```python
from build123d import *

# Parameters (mm, degrees)
F1_DEPTH = 12
F3_R     = 3


with BuildPart() as f1:
    # F0 (on Front) → F1 (new body)
    with BuildSketch(Plane.XZ):
        with BuildLine():
            Line((813.389391, 66.97586), (-386.610609, 66.97586))
            Line((-386.610609, 66.97586), (-386.610609, 26.97586))
            Line((-386.610609, 26.97586), (-406.610609, 26.97586))
            Line((-406.610609, 26.97586), (-406.610609, 11.97586))
            ThreePointArc((-406.610609, 11.97586), (-399.288279, -5.70181), (-381.610609, -13.02414))
            Line((-381.610609, -13.02414), (333.389391, -13.02414))
            ThreePointArc((333.389391, -13.02414), (351.06706, -5.70181), (358.389391, 11.97586))
            Line((358.389391, 11.97586), (658.389391, 11.97586))
            ThreePointArc((658.389391, 11.97586), (665.711721, -5.70181), (683.389391, -13.02414))
            Line((683.389391, -13.02414), (808.389391, -13.02414))
            ThreePointArc((808.389391, -13.02414), (826.06706, -5.70181), (833.389391, 11.97586))
            Line((833.389391, 11.97586), (833.389391, 26.97586))
            Line((833.389391, 26.97586), (813.389391, 26.97586))
            Line((813.389391, 26.97586), (813.389391, 66.97586))
        make_face()
    extrude(amount=F1_DEPTH)

    # F3
    f3_edges = [f1.edges().sort_by_distance(p)[0] for p in [
        (213.389391, -12, 66.97586),
        (-386.610609, -12, 46.97586),
        (-396.610609, -12, 26.97586),
        (-406.610609, -12, 19.47586),
        (-399.288279, -12, -5.70181),
        (-24.110609, -12, -13.02414),
        (351.06706, -12, -5.70181),
        (508.389391, -12, 11.97586),
        (665.711721, -12, -5.70181),
        (745.889391, -12, -13.02414),
        (826.06706, -12, -5.70181),
        (833.389391, -12, 19.47586),
        (823.389391, -12, 26.97586),
        (813.389391, -12, 46.97586),
        (213.389391, 0, 66.97586),
        (-386.610609, 0, 46.97586),
        (-396.610609, 0, 26.97586),
        (-406.610609, 0, 19.47586),
        (-399.288279, 0, -5.70181),
        (-24.110609, 0, -13.02414),
        (351.06706, 0, -5.70181),
        (508.389391, 0, 11.97586),
        (665.711721, 0, -5.70181),
        (745.889391, 0, -13.02414),
        (826.06706, 0, -5.70181),
        (833.389391, 0, 19.47586),
        (823.389391, 0, 26.97586),
        (813.389391, 0, 46.97586),
    ]]
    fillet(f3_edges, radius=F3_R)


solid = f1.part
```
The model under review builds one solid part; all positions refer to its coordinate system, in mm. A direction names the side the tool comes from. Give positions to 0.01 mm unless a question says otherwise; leave off trailing zeros. Loops run counter-clockwise (first coordinate to the right, second up) from the corner with the lowest first, then second, coordinate; pieces in that order, holes last. Notation, with made-up numbers: (-40, 60) -> (-34, 60) arc R27 cw to (-34, 78) -> close; hole circle Ø1 at (29, 56). An arc over 180 degrees is marked (long way). Use CSV: the item, a comma, the result in double quotes.
1. The part is to be moulded in two halves that separate along X. For faces 1 (the face through (205, 0, 27)), 2 (the face through (825.872, -5.958, -5.895)), 3 (the face through (665.52, -5.96, -5.51)), say which applies: +X half, -X half, draft (parallel to the pull), parting line (faces both ways), or undercut.
Result:
face 1,"draft"
face 2,"+X half"
face 3,"undercut"
2. For P1, Ø6.5, axis at x = 479, y = -7.5, coming from the -Z side; P2, Ø3, axis at y = -1.5, z = 58.5, coming from the -X side; P3, Ø5, axis at y = -6, z = 37, coming from the +X side, all flat-tipped, find the tip position at first contact; note any pin that passes through.
Result:
P1,"stops at z = 11.98"
P2,"stops at x = -386.61"
P3,"stops at x = 813.39"
3. Consider section C-C, the plane y = -6.5. Write out the cut boundary in (x, z), then the cut area to 3 significant figures.
Result:
outline,"(-406.61, 11.98) arc R25 ccw to (-381.61, -13.02) -> (333.39, -13.02) arc R25 ccw to (358.39, 11.98) -> (658.39, 11.98) arc R25 ccw to (683.39, -13.02) -> (808.39, -13.02) arc R25 ccw to (833.39, 11.98) -> (833.39, 26.98) -> (813.39, 26.98) -> (813.39, 66.98) -> (-386.61, 66.98) -> (-386.61, 26.98) -> (-406.61, 26.98) -> close"
area,"89,600 mm²"
4. Machinability: for faces 4 (the face through (205, -12, 27)), 5 (the face through (350.872, -5.958, -5.895)), which of the approach directions +Z, -Z, +X, -X, +Y, -Y give a long, thin tool a straight path to every point of the face, cutting with its end or side? Answer none if there is none.
Result:
face 4,"+Z, -Z, +X, -X, -Y"
face 5,"-Z, +Y, -Y"
5. Consider section A-A, the plane x = 507. Write out the cut boundary in (y, z), then the cut area to 3 significant figures.
Result:
outline,"(-12, 14.98) arc R3 ccw to (-9, 11.98) -> (-3, 11.98) arc R3 ccw to (0, 14.98) -> (0, 63.98) arc R3 ccw to (-3, 66.98) -> (-9, 66.98) arc R3 ccw to (-12, 63.98) -> close"
area,"652 mm²"
6. Consider section B-B, the plane z = 52.5. Write out the cut boundary in (x, y), then the cut area to 3 significant figures.
Result:
outline,"(-386.61, -9) arc R3 ccw to (-383.61, -12) -> (810.39, -12) arc R3 ccw to (813.39, -9) -> (813.39, -3) arc R3 ccw to (810.39, 0) -> (-383.61, 0) arc R3 ccw to (-386.61, -3) -> close"
area,"14,400 mm²"
7. To check wall thickness, follow probe 1 along X at (y, z) = (-6.5, 10); probe 2 along Z at (x, y) = (684, -9.75); probe 3 along X at (y, z) = (-4, 41.5). State the ranges of each line that lie inside material, in increasing order. Write a range as from..to.
Result:
probe 1,"x = -406.53..358.31, 658.47..833.31"
probe 2,"z = -12.93..66.88"
probe 3,"x = -386.61..813.39"
